Check sheet for the modelled part. Datum: model origin and axes. Units: mm. Give positions to 0.01 mm unless a question says otherwise; leave off trailing zeros. Loops run counter-clockwise (first coordinate to the right, second up) from the corner with the lowest first, then second, coordinate; pieces in that order, holes last. Notation, with made-up numbers: (-29.75, 7) -> (-19.75, 7) arc R16 cw to (-19.75, 12) -> close; hole circle Ø6 at (64, 70). An arc over 180 degrees is marked (long way). Answer as CSV lines item,"result". Start each with the question number.
(1) Gauge pin test, flat ends, axial feed: pin 1 Ø3 at (x, z) = (-10, 2.5) entering from +Y; pin 2 Ø1.2 at (x, z) = (0.5, 2.5) entering from -Y; pin 3 Ø2 at (y, z) = (5, 1) entering from -X. Record the tip position at first contact, or that the pin passes through.
(2) Section check B-B on z = 1.4. Enter the section's corners in (x, y).
(3) Section check A-A on y = 0. Enter the section's corners in (x, z), plus the area to 3 significant figures.
(4) Material ranges on line 1 (Y direction, x = -2, z = 2.5); line 2 (X direction, y = 10.5, z = 1.9); line 3 (X direction, y = -15, z = 0.4), recorded low to high. Write a range as from..to.
from build123d import *

# Parameters (mm, degrees)
F0_R     = 40
F0_W     = 5.02
F0_H     = 5.02
F1_DEPTH = 5
F2_R     = 0.45
F3_R     = 2


with BuildPart() as f1:
    # F0 (on Top) → F1 (new body)
    with BuildSketch(Plane.XY):
        Circle(F0_R)
        Rectangle(F0_W, F0_H, mode=Mode.SUBTRACT)
    extrude(amount=F1_DEPTH)

    # F2
    f2_edges = [f1.edges().sort_by_distance(p)[0] for p in [
        (-2.51, 2.51, 2.5),
        (-2.51, -2.51, 2.5),
        (2.51, -2.51, 2.5),
        (2.51, 2.51, 2.5),
    ]]
    fillet(f2_edges, radius=F2_R)

    # F3
    f3_edges = [f1.edges().sort_by_distance(p)[0] for p in [
        (-40, 0, 5),
    ]]
    fillet(f3_edges, radius=F3_R)


solid = f1.part
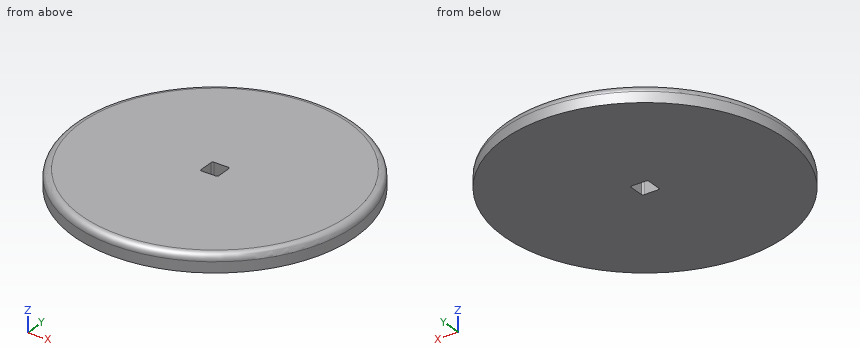
Working result:
1,pin 1,"stops at y = 39.09"
1,pin 2,"stops at y = -40"
1,pin 3,"stops at x = -39.8"
2,outline,"circle Ø80 at (0, 0); hole (-2.51, -2.06) arc R0.45 ccw to (-2.06, -2.51) -> (2.06, -2.51) arc R0.45 ccw to (2.51, -2.06) -> (2.51, 2.06) arc R0.45 ccw to (2.06, 2.51) -> (-2.06, 2.51) arc R0.45 ccw to (-2.51, 2.06) -> close"
3,outline,"(-40, 0) -> (-2.51, 0) -> (-2.51, 5) -> (-38, 5) arc R2 ccw to (-40, 3) -> close; (2.51, 0) -> (40, 0) -> (40, 3) arc R2 ccw to (38, 5) -> (2.51, 5) -> close"
3,area,"373 mm^2"
4,line 1,"y = -39.95..-2.51, 2.51..39.95"
4,line 2,"x = -38.6..38.6"
4,line 3,"x = -37.08..37.08"
